Geometry: final body of the model. Coordinates: model frame, mm. A direction names the side the tool comes from. Give positions to 0.01 mm unless a question says otherwise; leave off trailing zeros. Order: outer loops, then holes, each group sorted by start corner. A loop starts at its lowest first (then second) coordinate and runs counter-clockwise, first axis right, second up. Notation, with made-up numbers: (19.5, -31.5) - (36.5, -31.5) arc R18 cw to (36.5, -7.5) - close; hole circle Ø8 at (53.25, -22.5). An arc over 180 degrees is marked (long way). Use one line per item in the form item = value.
Autodesk Inventor part; units mm, degrees
ref_plane "Work Plane1" through (9, 0, 0) normal (1, 0, 0) x (0, 0, -1)
ref_plane "YZ Plane" through (0, 0, 0) normal (1, 0, 0) x (0, 1, 0)
ref_plane "XZ Plane" through (0, 0, 0) normal (0, 1, 0) x (-1, 0, 0)
sketch "Sketch1" plane through (0, 0, 0) normal (1, 0, 0) x (0, 1, 0)
  point P0 (0, 0)
sketch "Sketch2" plane through (0, 0, 0) normal (1, 0, 0) x (0, 1, 0)
  line L0 (15, 9) -> (-15, 9)
  line L1 (-15, 9) -> (-15, -9)
  line L2 (-15, -9) -> (15, -9)
  line L3 (15, -9) -> (15, 9)
  line L4 (15, 9) -> (-15, -9) construction
  line L5 (-15, 9) -> (15, -9) construction
  point P0 (0, 0)
  dimension "d0" = 30
  dimension "d1" = 18
extrude "Extrusion1" add sketch "Sketch2" along normal blind 18
sketch "Sketch3" plane through (0, -15, 9) normal (0, 0, 1) x (1, 0, 0)
  line L0 (18, 0) -> (18, 30)
  line L1 (0, 0) -> (0, 30)
  line L2 (18, 0) -> (0, 30)
  line L3 (0, 0) -> (18, 0)
  line L4 (0, 30) -> (0, 0)
  line L5 (0, 0) -> (18, 30)
  circle A0 centre (9, 15) radius 8.5
  point P0 (0, 15)
  dimension "d4" = 17
extrude "Extrusion2" add sketch "Sketch3" along normal blind 5 contours A0 L5 L2 | L2 L5 A0 | L5 L2 A0 | L5 A0 L2
sketch "Sketch4" plane through (9, 0, 14) normal (0, 0, 1) x (1, 0, 0)
  circle A0 centre (0, 0) radius 6
  point P0 (-9, 0)
  dimension "d7" = 12
extrude "Extrusion3" add sketch "Sketch4" along normal blind 7.5
sketch "Sketch5" plane through (9, 0, 21.5) normal (0, 0, 1) x (1, 0, 0)
  circle A0 centre (0, 0) radius 6
  point P0 (-9, 0)
extrude "Extrusion4" add sketch "Sketch5" along normal blind 5.5
sketch "Sketch6" plane through (0, 0, 0) normal (1, 0, 0) x (0, 1, 0)
  point P0 (0, 0)
ref_plane "Work Plane1" through (9, 0, 0) normal (1, 0, 0) x (0, 0, -1)
sketch "Sketch7" plane through (9, 0, 0) normal (1, 0, 0) x (0, 0, -1)
  line L0 (-27, 6) -> (-27, -6)
  line L1 (-27, 0) -> (-27, 3.7)
  line L2 (-27, 0) -> (-27, -3.7)
  line L3 (-14, -6) -> (-14, 6)
  line L4 (-14, -6) -> (-21.5, -6)
  line L5 (-14, -6) -> (-27, -6)
  line L6 (-21.5, -6) -> (-27, -3.7)
  line L7 (-27, -6) -> (-27, -3.7)
  line L8 (-21.5, -6) -> (-27, -6)
  line L9 (-40.6184, 0) -> (-19.5493, 0)
  point P0 (0, 0)
  dimension "d12" = 3.7
  dimension "d13" = 3.7
  dimension "d14" = 7.5
revolve "Revolution1" cut sketch "Sketch7" angle 360 about axis through (9, 0, 40.6184) along (0, 0, -1)
sketch "Sketch8" plane through (9, 0, 27) normal (0, 0, 1) x (1, 0, 0)
  circle A0 centre (0, 0) radius 3.7
  circle A1 centre (0, 0) radius 5.35
  point P0 (-9, 0)
  dimension "d16" = 10.7
extrude "Extrusion5" add sketch "Sketch8" along normal blind 26.4 contours A0 | A1
sketch "Sketch9" plane through (9, 0, 0) normal (1, 0, 0) x (0, 0, -1)
  line L0 (-27, 3.7) -> (-27, -3.7)
  line L1 (-27, 3.7) -> (-53.4, 5.35)
  line L2 (-27, 5.35) -> (-53.4, 5.35)
  line L3 (-27, 3.7) -> (-27, 5.35)
  line L4 (-66.1655, 0) -> (-43.0091, 0)
  line L5 (-53.4, 5.35) -> (-53.4, -5.35)
  point P0 (0, 0)
  point P1 (-53.4, 0)
revolve "Revolution2" cut sketch "Sketch9" angle 360 about axis through (9, 0, 66.1655) along (0, 0, -1)
thread "Thread1"
properties part number "NKK_S1AL" material "Stainless Steel"
(1) Reachability of faces 1 (the face through (9, -15, 0)), 2 (the face through (2.735, -5.745, 11.465)) from +Z, -Z, +X, -X, +Y, -Y: full face, straight path, thin tool, end or side. Return the list, or none.
Computed values:
face_1 = +Z, -Z, +X, -X, -Y
face_2 = +Z
(2) Pull-direction query (Z, two-part tool) for faces 3 (the face through (18, 0, 0)), 4 (the face through (13.025, 2.093, 40.385)), 5 (the face through (9, 0, -9)), 6 (the face through (13.002, 0.889, 26.045)); classes: released by +Z, released by -Z, zero draft, split by the parting line, or undercut.
Computed values:
face_3 = zero draft
face_4 = undercut
face_5 = released by -Z
face_6 = undercut
(3) Cut plane D-D on x = 1.75. Output: boundary loops of the cut face in (y, z).
Computed values:
outline = (-15, -9) - (15, -9) - (15, 9) - (4.44, 9) - (4.44, 14) - (-4.44, 14) - (-4.44, 9) - (-15, 9) - close
(4) Contact query for flat-ended pins moving along their axis: pin 1 Ø1.5 at (x, z) = (8.5, 29) entering from -Y; pin 2 Ø6 at (x, z) = (11.5, 40.5) entering from +Y; pin 3 Ø10 at (y, z) = (-3, 43.5) entering from -X. Output: stop coordinate, or through.
Computed values:
pin_1 = -3.86
pin_2 = 4.66
pin_3 = 4.01
(5) Cut plane B-B on x = 9. Output: boundary loops of the cut face in (y, z).
Computed values:
outline = (-15, -9) - (15, -9) - (15, 9) - (8.5, 9) - (8.5, 14) - (6, 14) - (6, 21.5) - (3.7, 27) - (5.35, 53.4) - (-5.35, 53.4) - (-3.7, 27) - (-6, 21.5) - (-6, 14) - (-8.5, 14) - (-8.5, 9) - (-15, 9) - close
(6) Cut plane C-C on z = 13. Output: boundary loops of the cut face in (x, y).
Computed values:
outline = circle Ø17 at (9, 0)
(7) Ray query, line 1 along Z through (x, y) = (4.75, -13.5); line 2 along Z through (x, y) = (5, 5.25); line 3 along X through (y, z) = (1, 50.5). Return the intervals inside material, ascending.
Computed values:
line_1 = -9 to 9
line_2 = -9 to 14
line_3 = 3.93 to 14.07
(8) Cut plane A-A on y = 0. Output: boundary loops of the cut face in (x, z), plus the area to 3 significant figures.
Computed values:
outline = (0, -9) - (18, -9) - (18, 9) - (17.5, 9) - (17.5, 14) - (15, 14) - (15, 21.5) - (12.7, 27) - (14.35, 53.4) - (3.65, 53.4) - (5.3, 27) - (3, 21.5) - (3, 14) - (0.5, 14) - (0.5, 9) - (0, 9) - close
area = 791 mm²
